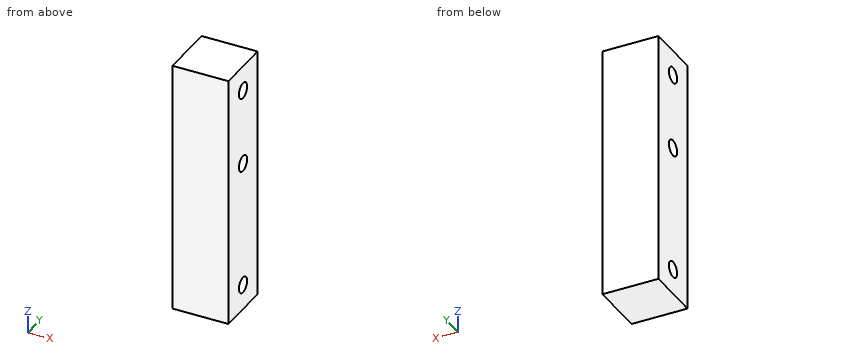
from build123d import *

# Parameters (mm, degrees)
SKETCH1_W           = 63.5
SKETCH1_H           = 13.97
BOSS_EXTRUDE3_DEPTH = 13.97
SKETCH3_R           = 1.9685
CUT_EXTRUDE1_DEPTH  = 254
SKETCH4_R           = 1.9685
CUT_EXTRUDE3_DEPTH  = 254


with BuildPart() as part:
    # Sketch1 → Boss-Extrude3 (new body)
    with BuildSketch(Plane(origin=(0, 0, 0), x_dir=(0, 0, -1), z_dir=(1, 0, 0))):
        with Locations((31.75, 6.985)):
            Rectangle(SKETCH1_W, SKETCH1_H)
    extrude(amount=BOSS_EXTRUDE3_DEPTH)

    # Sketch3 → Cut-Extrude1 (cut)
    with BuildSketch(Plane(origin=(13.97, 0, 0), x_dir=(0, 0, -1), z_dir=(1, 0, 0))):
        with Locations((6.35, 6.985)):
            Circle(SKETCH3_R)
        with Locations((57.15, 6.985)):
            Circle(SKETCH3_R)
    extrude(amount=-CUT_EXTRUDE1_DEPTH, mode=Mode.SUBTRACT)

    # Sketch4 → Cut-Extrude3 (cut)
    with BuildSketch(Plane(origin=(13.97, 0, 0), x_dir=(0, 0, -1), z_dir=(1, 0, 0))):
        with Locations((25.4, 6.985)):
            Circle(SKETCH4_R)
    extrude(amount=-CUT_EXTRUDE3_DEPTH, mode=Mode.SUBTRACT)


solid = part.part
Can you work these out from the model? Positions are in its coordinate system, mm. Coordinates: 2 decimals unless noted, no trailing zeros. Loops run counter-clockwise (first coordinate to the right, second up) from the corner with the lowest first, then second, coordinate; pieces in that order, holes last. Notation, with made-up numbers: M 86.5,49 L 107.5,49 A22 ccw 107.5,72 Z; hole C -33,56.25 d7. An arc over 180 degrees is marked long. Return JSON: item names as keys, results as strings. Group by question number.
Item 1: Imagine slicing it at B-B (y = 6.25). Please give me the cut outline in (x, z), and give its area (3 significant figures).
Item 2: If I drill on L1, parallel to Y at x = 10.5, z = -6.35; L2, parallel to Z at x = 6, y = 8.75; L3, parallel to Z at x = 11.25, y = 5.75, over which ranges is the centre line in solid material (lowest first)? Write a range as from..to.
Item 3: I'm going to push flat-ended pins straight in: pin 1 Ø4 at (y, z) = (7, -30.5) entering from -X; pin 2 Ø3 at (y, z) = (6.985, -57.15) entering from -X. Where does each tip first touch, or does it pass through?
Item 4: Imagine slicing it at C-C (x = 8.75). Give the number of separate pieces and of enclosed holes in the cut face, and give its area (3 significant figures).
Item 5: Imagine slicing it at A-A (z = -57.15). Please give me the cut outline in (x, y), and give its area (3 significant figures).
Verdict:
{
 "1": {"outline": "M 0,-63.5 L 13.97,-63.5 L 13.97,-58.98 L 0,-58.98 Z; M 0,-55.32 L 13.97,-55.32 L 13.97,-27.23 L 0,-27.23 Z; M 0,-23.57 L 13.97,-23.57 L 13.97,-8.18 L 0,-8.18 Z; M 0,-4.52 L 13.97,-4.52 L 13.97,0 L 0,0 Z", "area": "734 mm^2"},
 "2": {"L1": "y = 0..5.02, 8.95..13.97", "L2": "z = -63.5..-58.02, -56.28..-26.27, -24.53..-7.22, -5.48..0", "L3": "z = -63.5..-58.68, -55.62..-26.93, -23.87..-7.88, -4.82..0"},
 "3": {"pin 1": "stops at x = 0", "pin 2": "passes through"},
 "4": {"separate pieces": "1", "enclosed holes": "3", "area": "851 mm^2"},
 "5": {"outline": "M 0,0 L 13.97,0 L 13.97,5.02 L 0,5.02 Z; M 0,8.95 L 13.97,8.95 L 13.97,13.97 L 0,13.97 Z", "area": "140 mm^2"}
}
